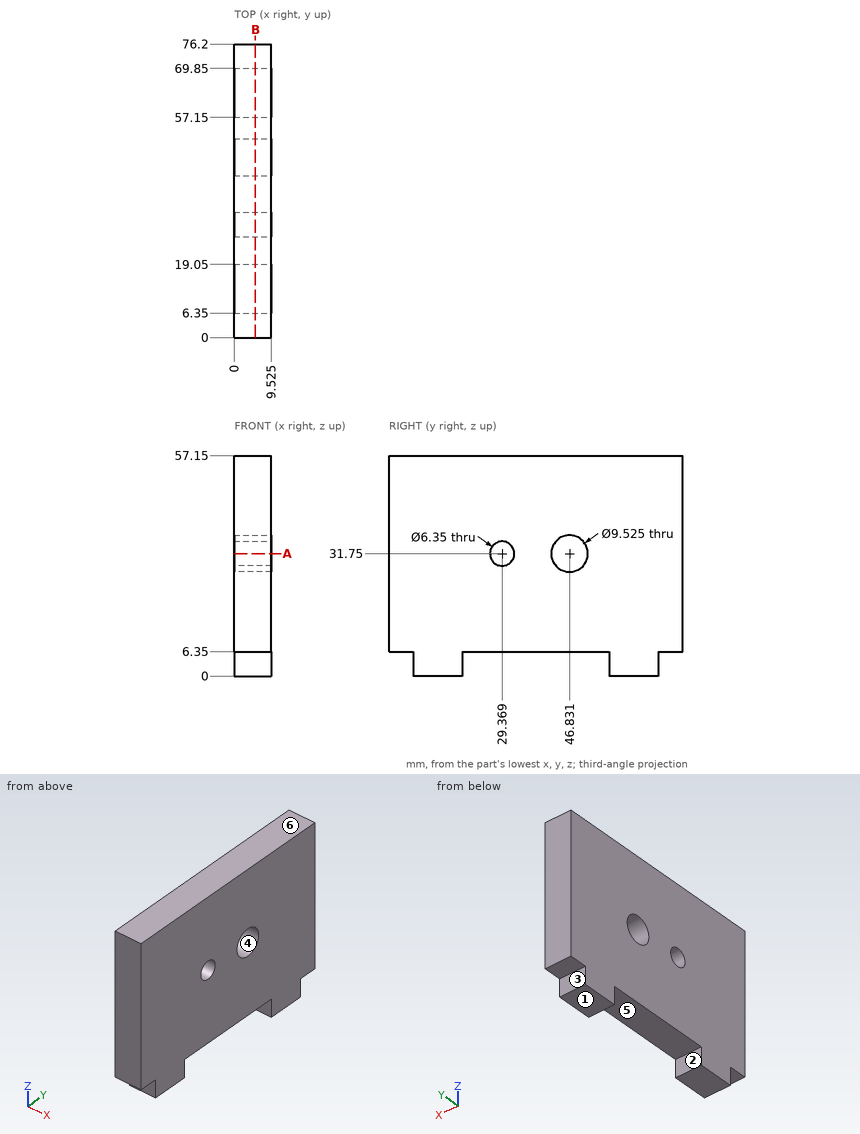
Design review of the part shown in the three views and the two pictorial views. Dimensions are in mm from the part's minimum x, y and z. A direction names the side the tool comes from. Round coordinates to 2 decimals unless told otherwise and drop trailing zeros. Write each loop counter-clockwise with the first axis right and the second up, starting at its lowest first coordinate (ties: lowest second). Pieces come first, ordered by that corner, then holes. Notation, with made-up numbers: (-4.75, 13) - (32.25, 13) arc R19 ccw to (32.25, 42) - close; hole circle Ø2 at (55, -28.5). An arc over 180 degrees is marked (long way). Write item = value, one per line. Start each with the question number.
1. Consider section B-B on x = 5.5. Give the number of separate pieces and of enclosed holes in the cut face, plus the area to 3 significant figures.
2. Consider section A-A on z = 31.75. State the section outline as (x, y) points (1 decimal), plus the area to 3 significant figures.
3. Draft analysis for pull direction Z (two halves, no side actions). For the marked faces 3, 4, 5 and 6, state which applies: released by +Z, released by -Z, zero draft, split by the parting line, or undercut.
4. Wall thickness on L1, parallel to Y at x = 7.25, z = 31.75; L2, parallel to Z at x = 3.75, y = 57; L3, parallel to Y at x = 2.25, z = 27.5: over which ranges is each line inside the solid? List them lowest first.
5. For pin 1 Ø3 at (x, y) = (5, 2.5) entering from -Z; pin 2 Ø5 at (x, z) = (6, 2.5) entering from +Y; pin 3 Ø3 at (x, z) = (5.5, 4.5) entering from -Y; pin 4 Ø5 at (y, z) = (29.37, 31.75) entering from +X, all flat-tipped, find the tip position at first contact; note any pin that passes through.
6. For the marked faces 1 and 2, list the 3-axis set-ups (+Z, -Z, +X, -X, +Y, -Y) from which the entire face can be reached by the end or side of a thin tool; tool diameter is ignored.
Evaluation:
q1.separate_pieces = 1
q1.enclosed_holes = 2
q1.area = 3,930 mm2
q2.outline = (0, 0) - (9.5, 0) - (9.5, 26.2) - (0, 26.2) - close; (0, 32.5) - (9.5, 32.5) - (9.5, 42.1) - (0, 42.1) - close; (0, 51.6) - (9.5, 51.6) - (9.5, 76.2) - (0, 76.2) - close
q2.area = 575 mm2
q3.face_3 = zero draft
q3.face_4 = undercut
q3.face_5 = released by -Z
q3.face_6 = released by +Z
q4.L1 = 0 to 26.19, 32.54 to 42.07, 51.59 to 76.2
q4.L2 = 6.35 to 57.15
q4.L3 = 0 to 44.68, 48.98 to 76.2
q5.pin_1 = 6.35
q5.pin_2 = 69.85
q5.pin_3 = 6.35
q5.pin_4 = through
q6.face_1 = -Z, +X, -X, +Y, -Y
q6.face_2 = -Z, +X, -X
